```python
from build123d import *

# Parameters (mm, degrees)
SKETCH1_W                = 12.5
SKETCH1_H                = 5.842
BOSS_EXTRUDE2_DEPTH      = 5.842
F_0_257_DIAMETER_HOLE1_D = 6.5278
SKETCH4_W                = 3.175
SKETCH4_H                = 8.0375
SKETCH4_H_2              = 6.35
CUT_EXTRUDE1_DEPTH       = 60.128735202


with BuildPart() as part:
    # Sketch1 → Boss-Extrude2 (new body)
    with BuildSketch(Plane(origin=(0, 0, 0), x_dir=(1, 0, 0), z_dir=(0, 1, 0))):
        with BuildLine():
            Line((0, 0), (-6.45, 0))
            Line((-6.45, 0), (-6.45, -5.842))
            Line((-6.45, -5.842), (-19.35, -5.842))
            Line((-19.35, -5.842), (-19.35, 0))
            Line((-19.35, 0), (-31.85, 0))
            Line((-31.85, 0), (-31.85, -5.842))
            Line((-31.85, -5.842), (-44.75, -5.842))
            Line((-44.75, -5.842), (-44.75, 0))
            Line((-44.75, 0), (-50.8, 0))
            Line((-50.8, 0), (-50.8, 8.0375))
            Line((-50.8, 8.0375), (-44.75, 8.0375))
            Line((-44.75, 8.0375), (-44.75, 13.8795))
            Line((-44.75, 13.8795), (-50.8, 13.8795))
            Line((-50.8, 13.8795), (-50.8, 17.0545))
            Line((-50.8, 17.0545), (-29.639726031, 28.654387599))
            ThreePointArc((-29.639726031, 28.654387599), (-25.6, 29.689027646), (-21.560273969, 28.654387599))
            Line((-21.560273969, 28.654387599), (-0.4, 17.0545))
            Line((-0.4, 17.0545), (-0.4, 13.8795))
            Line((-0.4, 13.8795), (-6.45, 13.8795))
            Line((-6.45, 13.8795), (-6.45, 8.0375))
            Line((-6.45, 8.0375), (0, 8.0375))
            Line((0, 8.0375), (0, 0))
        make_face()
        with Locations((-25.6, 10.9585)):
            Rectangle(SKETCH1_W, SKETCH1_H, mode=Mode.SUBTRACT)
    extrude(amount=BOSS_EXTRUDE2_DEPTH)

    # F (0.257) Diameter Hole1 (through all)
    with Locations(Plane(origin=(0, 5.842, 0), x_dir=(1, 0, 0), z_dir=(0, 1, 0))):
        with Locations((-25.6, 23.339027646)):
            Hole(F_0_257_DIAMETER_HOLE1_D / 2)

    # Sketch4 → Cut-Extrude1 (cut, through all)
    with BuildSketch(Plane(origin=(0, 5.842, 0), x_dir=(1, 0, 0), z_dir=(0, 1, 0))):
        with Locations((-49.2125, 4.01875)):
            Rectangle(SKETCH4_W, SKETCH4_H)
        Polygon((-3.575, 9.495445591), (-3.575, 0), (-0.4, 0), (0, 0), (0, 9.495445591), (-0.4, 9.495445591), align=None)
        with Locations((-49.2125, 17.0545)):
            Rectangle(SKETCH4_W, SKETCH4_H_2)
        with Locations((-1.9875, 16.9545)):
            Rectangle(SKETCH4_W, SKETCH4_H_2)
    extrude(amount=-CUT_EXTRUDE1_DEPTH, mode=Mode.SUBTRACT)


solid = part.part
```
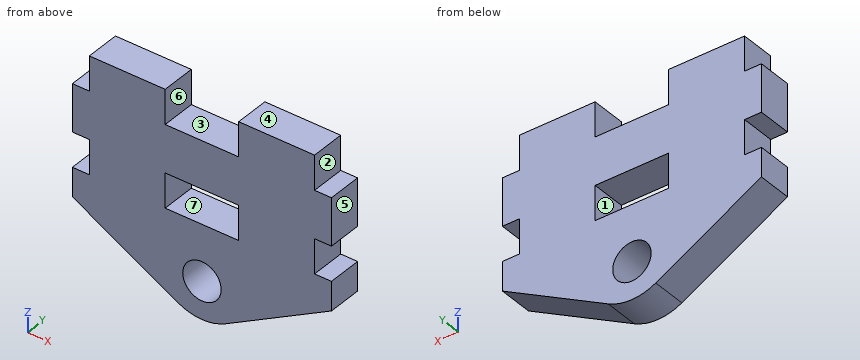
Build history of the part. All positions in model axes, mm. Face numbers are marked on the shaded views. A direction names the side the tool comes from. Round coordinates to 2 decimals unless told otherwise and drop trailing zeros. Loops run counter-clockwise (first coordinate to the right, second up) from the corner with the lowest first, then second, coordinate; pieces in that order, holes last.
Item 1: Saw through at A-A (z = -9). List the corners of the cut face in (x, y).
Item 2: Saw through at D-D (x = -44). List the corners of the cut face in (y, z).
Item 3: Pin check, flat tips, straight feed: P1, Ø1, axis at x = -10, y = 1, coming from the -Z side; P2, Ø4, axis at x = -25.6, z = -23.34, coming from the +Y side; P3, Ø1.8, axis at y = 3.5, z = -11, coming from the -X side; P4, Ø3, axis at x = -45.5, y = 2.5, coming from the +Z side. Stop position of each tip, or through.
Item 4: Which spindle directions (+Z, -Z, +X, -X, +Y, -Y) get a long thin tool onto all of the face, cutting with end or side? Do the marked faces 1, 2 and 3. Say none if no direction does.
Item 5: Saw through at C-C (y = 1.6). State how many separate pieces and enclosed holes the cut face has, then the cut area to 3 significant figures.
Item 6: Two-plate mould, pull along X, no slides. Class the marked faces 4, 5, 6 and 7: released by +X, released by -X, zero draft, split by the parting line, or undercut.
Item 7: Saw through at B-B (x = -25.6). List the corners of the cut face in (y, z).
Item 8: Drill centre lines: line 1 along Z through (x, y) = (-25.6, 1.6); line 2 along X through (y, z) = (1.8, 0.5); line 3 along Z through (x, y) = (-28, 3.95). Where is each one in solid material? Low to high.
Worked answers:
1. outline: (-44.75, 0) - (-31.85, 0) - (-31.85, 5.84) - (-44.75, 5.84) - close; (-19.35, 0) - (-6.45, 0) - (-6.45, 5.84) - (-19.35, 5.84) - close
2. outline: (0, -20.78) - (5.84, -20.78) - (5.84, 5.84) - (0, 5.84) - close
3. P1: stops at z = -22.59
3. P2: passes through
3. P3: stops at x = -44.75
3. P4: stops at z = 5.84
4. face 1: +Y, -Y
4. face 2: +Z, +X, +Y, -Y
4. face 3: +Z, +Y, -Y
5. separate pieces: 1
5. enclosed holes: 2
5. area: 1,100 mm2
6. face 4: zero draft
6. face 5: released by +X
6. face 6: undercut
6. face 7: undercut
7. outline: (0, -29.69) - (5.84, -29.69) - (5.84, -26.6) - (0, -26.6) - close; (0, -20.08) - (5.84, -20.08) - (5.84, -13.88) - (0, -13.88) - close; (0, -8.04) - (5.84, -8.04) - (5.84, 0) - (0, 0) - close
8. line 1: z = -29.69 to -26.6, -20.08 to -13.88, -8.04 to 0
8. line 2: x = -44.75 to -31.85, -19.35 to -6.45
8. line 3: z = -29.34 to -25.55, -21.13 to -13.88, -8.04 to 0
